Input: dimensioned drawing with shaded views. Units: mm. Origin: part minimum x, y, z. Give positions to 0.01 mm unless a question says otherwise; leave off trailing zeros. Order: outer loops, then holes, each group sorted by start corner. A loop starts at its lowest first (then second) coordinate and runs counter-clockwise, first axis right, second up.
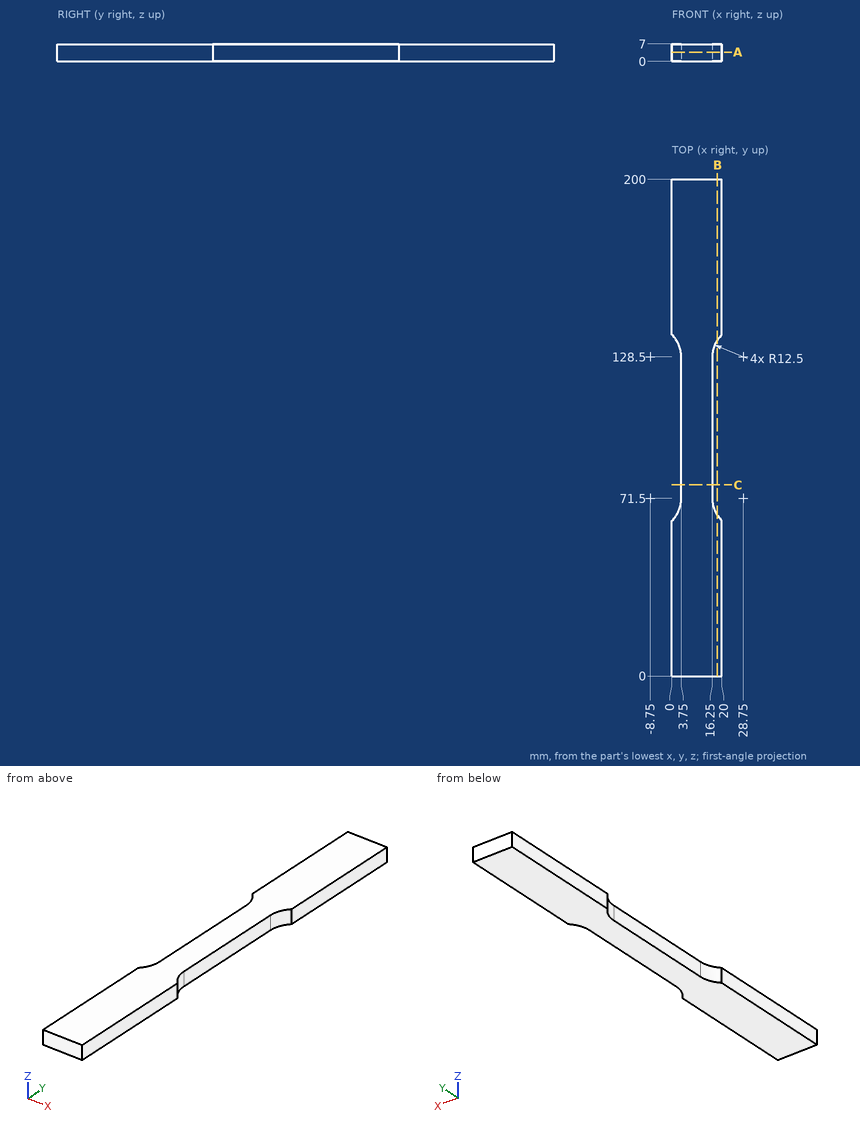
1) Material intervals for L1, parallel to X at y = 104, z = 5; L2, parallel to Y at x = 17.5, z = 1, sorted ascending.
Report:
L1: x = 3.75 to 16.25
L2: y = 0 to 66.05, 133.95 to 200
2) Section query C-C, the plane y = 77. Return the cut outline in (x, z).
Report:
outline: (3.75, 0) - (16.25, 0) - (16.25, 7) - (3.75, 7) - close
3) Section query B-B, the plane x = 18.25. Return the cut outline in (y, z), and give its area (3 significant figures).
Report:
outline: (0, 0) - (64.72, 0) - (64.72, 7) - (0, 7) - close; (135.28, 0) - (200, 0) - (200, 7) - (135.28, 7) - close
area: 906 mm2
4) Section query A-A, the plane z = 3.75. Return the cut outline in (x, y), and give its area (3 significant figures).
Report:
outline: (0, 0) - (20, 0) - (20, 62.57) arc R12.5 cw to (16.25, 71.5) - (16.25, 128.5) arc R12.5 cw to (20, 137.43) - (20, 200) - (0, 200) - (0, 137.43) arc R12.5 cw to (3.75, 128.5) - (3.75, 71.5) arc R12.5 cw to (0, 62.57) - close
area: 3,480 mm2
